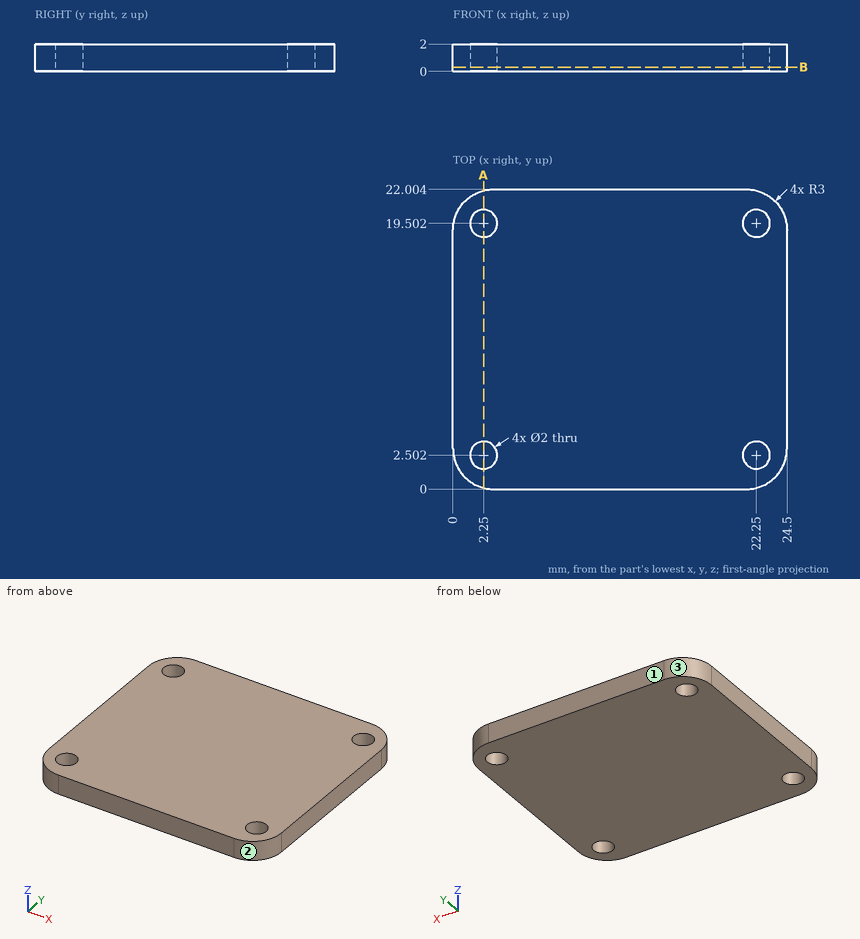
Input: dimensioned drawing with shaded views. Units: mm. Origin: part minimum x, y, z. Coordinates: 2 decimals unless noted, no trailing zeros. Order: outer loops, then holes, each group sorted by start corner. A loop starts at its lowest first (then second) coordinate and runs counter-clockwise, first axis right, second up. Notation, with made-up numbers: (-8, -27) - (-1, -27) arc R20 ccw to (-1, -3) - close; hole circle Ø3 at (25.5, -7). An arc over 180 degrees is marked (long way). Return JSON: item names as keys, results as strings. Group by question number.
1. Material intervals for line 1 along Y through (x, z) = (22.25, 1.3) (1 decimal); line 2 along X through (y, z) = (20.25, 0.3); line 3 along Y through (x, z) = (23.5, 1.4) (1 decimal), sorted ascending. Write a range as [from, to].
2. Cut plane B-B (z = 0.3). Output: boundary loops of the cut face in (x, y), plus the area to 3 significant figures.
3. Pull-direction query (X, two-part tool) for the marked faces 1, 2 and 3; classes: pulls with the +X half, pulls with the -X half, needs draft (parallel to the pull), parting line crosses it, or undercut.
4. Cut plane A-A (x = 2.25). Output: boundary loops of the cut face in (y, z) (1 decimal).
Resolved:
{
 "1": {"line 1": "y = [0.1, 1.5], [3.5, 18.5], [20.5, 21.9]", "line 2": "x = [0.27, 1.59], [2.91, 21.59], [22.91, 24.23]", "line 3": "y = [0.8, 21.2]"},
 "2": {"outline": "(0, 3) arc R3 ccw to (3, 0) - (21.5, 0) arc R3 ccw to (24.5, 3) - (24.5, 19) arc R3 ccw to (21.5, 22) - (3, 22) arc R3 ccw to (0, 19) - close; hole circle Ø2 at (2.25, 2.5); hole circle Ø2 at (2.25, 19.5); hole circle Ø2 at (22.25, 2.5); hole circle Ø2 at (22.25, 19.5)", "area": "519 mm²"},
 "3": {"face 1": "needs draft", "face 2": "pulls with the +X half", "face 3": "pulls with the -X half"},
 "4": {"outline": "(0.1, 0) - (1.5, 0) - (1.5, 2) - (0.1, 2) - close; (3.5, 0) - (18.5, 0) - (18.5, 2) - (3.5, 2) - close; (20.5, 0) - (21.9, 0) - (21.9, 2) - (20.5, 2) - close"}
}
